Input: dimensioned drawing with shaded views. Units: mm. Origin: part minimum x, y, z. A direction names the side the tool comes from. Give positions to 0.01 mm unless a question says otherwise; leave off trailing zeros. Write each loop counter-clockwise with the first axis right and the second up, starting at its lowest first coordinate (ties: lowest second). Pieces come first, ordered by that corner, then holes. Notation, with made-up numbers: M 33.25,13 L 77.25,13 A32 cw 77.25,50 Z; hole C 58,82.25 d5. An arc over 180 degrees is marked long. Use CSV: the item, a comma, the result in double quotes. Start each with the question number.
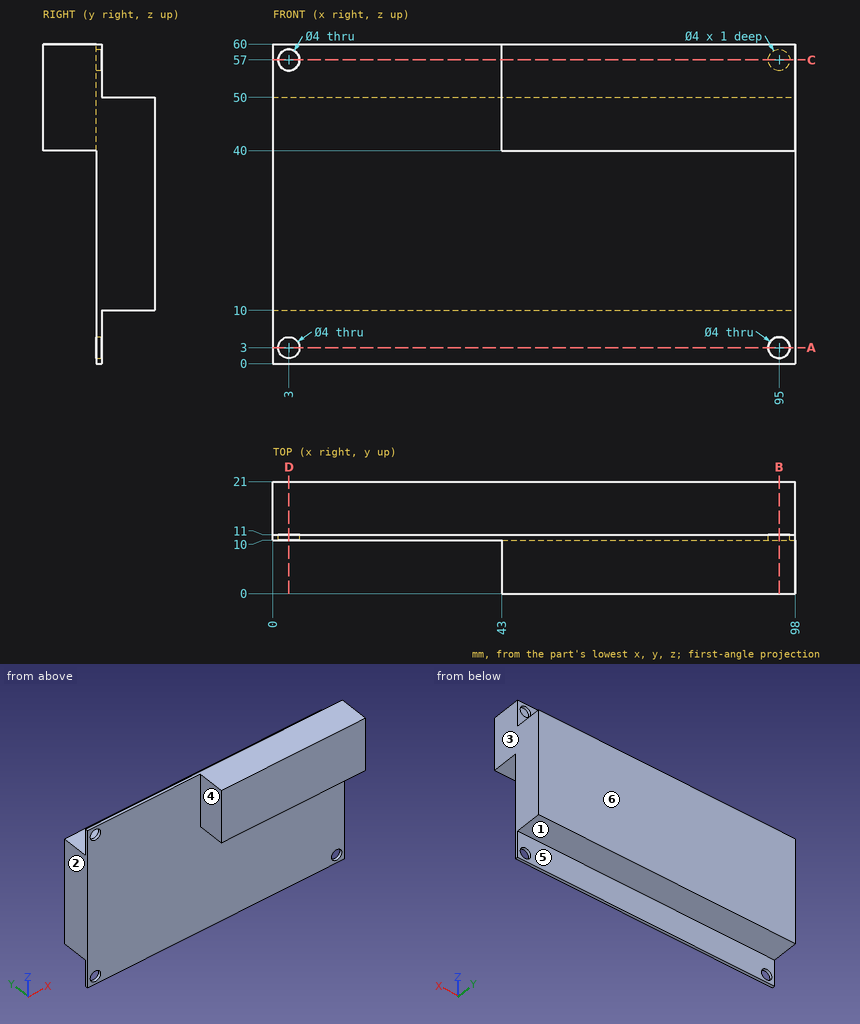
Q1. Set-up query: the marked faces 4, 5 and 6. Return all of +Z, -Z, +X, -X, +Y, -Y with unobstructed straight access to the full face (end or side cutting, diameter ignored); none if empty.
Q2. Section C-C, the plane z = 57. Return the cut outline in (x, y), and give its area (3 significant figures).
Q3. Section A-A, the plane z = 3. Return the cut outline in (x, y).
Q4. Pull-direction query (X, two-part tool) for the marked faces 1, 2 and 3; classes: released by +X, released by -X, zero draft, split by the parting line, or undercut.
Q5. Material intervals for L1, parallel to X at y = 10.5, z = 3; L2, parallel to Z at x = 95, y = 10.7; L3, parallel to Y at x = 36.5, z = 13, sorted ascending. Write a range as [from, to].
Q6. Section D-D, the plane x = 3. Return the cut outline in (y, z).
Q7. Section B-B, the plane x = 95. Return the cut outline in (y, z), and give its area (3 significant figures).
Q8. First-contact query: pin 1 Ø4 at (x, y) = (21.5, 16.5) entering from +Z; pin 2 Ø2 at (x, z) = (95, 57) entering from +Y; pin 3 Ø5 at (x, z) = (3, 3) entering from -Y. Flat tips, straight axial feed; report the tip coordinate or a pass-through.
Check result:
1,face 4,"+Z, -Z, -X, -Y"
1,face 5,"-Z, +X, -X, +Y"
1,face 6,"+Z, -Z, +X, -X, +Y"
2,outline,"M 0,10 L 1,10 L 1,11 L 0,11 Z; M 5,10 L 43,10 L 43,0 L 98,0 L 98,11 L 97,11 L 97,10 L 93,10 L 93,11 L 5,11 Z"
2,area,"640 mm²"
3,outline,"M 0,10 L 1,10 L 1,11 L 0,11 Z; M 5,10 L 93,10 L 93,11 L 5,11 Z; M 97,10 L 98,10 L 98,11 L 97,11 Z"
4,face 1,"zero draft"
4,face 2,"released by -X"
4,face 3,"released by +X"
5,L1,"x = [0, 1], [5, 93], [97, 98]"
5,L2,"z = [0, 1], [5, 55], [59, 60]"
5,L3,"y = [10, 21]"
6,outline,"M 10,0 L 11,0 L 11,1 L 10,1 Z; M 10,5 L 11,5 L 11,10 L 21,10 L 21,50 L 11,50 L 11,55 L 10,55 Z; M 10,59 L 11,59 L 11,60 L 10,60 Z"
7,outline,"M 0,40 L 10,40 L 10,5 L 11,5 L 11,10 L 21,10 L 21,50 L 11,50 L 11,55 L 10,55 L 10,59 L 11,59 L 11,60 L 0,60 Z; M 10,0 L 11,0 L 11,1 L 10,1 Z"
7,area,"652 mm²"
8,pin 1,"stops at z = 50"
8,pin 2,"stops at y = 10"
8,pin 3,"stops at y = 10"
